Here's how the part is built. I have some questions about the finished solid (model axes, mm). Face numbers are marked on the shaded views. A direction names the side the tool comes from. Coordinates: 2 decimals unless noted, no trailing zeros. Write each loop counter-clockwise with the first axis right and the second up, starting at its lowest first coordinate (ties: lowest second). Pieces come first, ordered by that corner, then holes.
Item 1: Please list where these lines run through material, in increasing order: line 1 (Z direction, x = 16, y = 0.35); line 2 (X direction, y = 6.5, z = 10); line 3 (Y direction, x = -16.5, z = 5).
Item 2: I want a section at C-C (y = 5.75). Please give me the cut outline in (x, z).
Item 3: I want a section at B-B (x = 0). Please give me the cut outline in (y, z), and give its area (3 significant figures).
Item 4: For the marked faces 1 and 2, which set-ups out of +Z, -Z, +X, -X, +Y, -Y let a thin tool reach every point of the face, with its end or its side?
Item 5: I want a section at D-D (z = 16). Count the separate pieces of the cut face and the enclosed holes in it, and give its area (3 significant figures).
Item 6: I'm going to push flat-ended pins straight in: P1, Ø4.5, axis at x = 16, z = 16, coming from the +Y side; P2, Ø6.5, axis at x = -16, z = 16, coming from the +Y side; P3, Ø1, axis at y = 7, z = 5.5, coming from the +X side; P4, Ø10, axis at x = 11, z = -9.5, coming from the -Y side. Where does each tip first touch, or does it pass through?
Item 7: I want a section at A-A (z = 0). Please give me the cut outline in (x, y), and give its area (3 significant figures).
from build123d import *

# Parameters (mm, degrees)
ESQUISSE1_W             = 42
ESQUISSE1_H             = 42
BOSS_EXTRU_1_DEPTH      = 1
CONG_1_R                = 3
ENL_V_MAT_EXTRU_1_REACH = 11
ESQUISSE3_R             = 2


with BuildPart() as part:
    # Esquisse1 → Boss.-Extru.1 (new body)
    with BuildSketch(Plane(origin=(0, 0, 0), x_dir=(1, 0, 0), z_dir=(0, 1, 0))):
        Rectangle(ESQUISSE1_W, ESQUISSE1_H)
    extrude(amount=BOSS_EXTRU_1_DEPTH)

    # Congé1
    cong_1_edges = [part.edges().sort_by_distance(p)[0] for p in [
        (-21, 0.5, -21),
        (21, 0.5, -21),
        (21, 0.5, 21),
        (-21, 0.5, 21),
    ]]
    fillet(cong_1_edges, radius=CONG_1_R)

    # Esquisse2 → Révolution1 (revolve)
    with BuildSketch(Plane(origin=(0, 0, 0), x_dir=(0, 0, -1), z_dir=(1, 0, 0))):
        with BuildLine():
            Line((-20, 1), (-16.490388922, 3.457456133))
            ThreePointArc((-16.490388922, 3.457456133), (-15.671777012, 3.861150852), (-14.769659613, 4))
            Line((-14.769659613, 4), (-14, 4))
            Line((-14, 4), (-14, 7))
            ThreePointArc((-14, 7), (-13.414213562, 8.414213562), (-12, 9))
            Line((-12, 9), (0, 9))
            Line((0, 9), (0, 4))
            Line((0, 4), (0, 1))
            Line((0, 1), (-20, 1))
        make_face()
    revolve(axis=Axis((0, 4, 0), (0, -1, 0)))

    # Esquisse3 → Enlèv. mat.-Extru.1 (cut, up to next)
    with BuildSketch(Plane.XZ, mode=Mode.PRIVATE) as enl_v_mat_extru_1_sk1:
        with Locations((-16, 16)):
            Circle(ESQUISSE3_R)
    enl_v_mat_extru_1_tool1 = extrude(enl_v_mat_extru_1_sk1.sketch, amount=-ENL_V_MAT_EXTRU_1_REACH, mode=Mode.PRIVATE) & part.part
    add(enl_v_mat_extru_1_tool1.solids().sort_by_distance((-16, 0, 16))[0], mode=Mode.SUBTRACT)
    # Esquisse3 → Enlèv. mat.-Extru.1 (cut, up to next)
    with BuildSketch(Plane.XZ, mode=Mode.PRIVATE) as enl_v_mat_extru_1_sk2:
        with Locations((16, 16)):
            Circle(ESQUISSE3_R)
    enl_v_mat_extru_1_tool2 = extrude(enl_v_mat_extru_1_sk2.sketch, amount=-ENL_V_MAT_EXTRU_1_REACH, mode=Mode.PRIVATE) & part.part
    add(enl_v_mat_extru_1_tool2.solids().sort_by_distance((16, 0, 16))[0], mode=Mode.SUBTRACT)
    # Esquisse3 → Enlèv. mat.-Extru.1 (cut, up to next)
    with BuildSketch(Plane.XZ, mode=Mode.PRIVATE) as enl_v_mat_extru_1_sk3:
        with Locations((-16, -16)):
            Circle(ESQUISSE3_R)
    enl_v_mat_extru_1_tool3 = extrude(enl_v_mat_extru_1_sk3.sketch, amount=-ENL_V_MAT_EXTRU_1_REACH, mode=Mode.PRIVATE) & part.part
    add(enl_v_mat_extru_1_tool3.solids().sort_by_distance((-16, 0, -16))[0], mode=Mode.SUBTRACT)
    # Esquisse3 → Enlèv. mat.-Extru.1 (cut, up to next)
    with BuildSketch(Plane.XZ, mode=Mode.PRIVATE) as enl_v_mat_extru_1_sk4:
        with Locations((16, -16)):
            Circle(ESQUISSE3_R)
    enl_v_mat_extru_1_tool4 = extrude(enl_v_mat_extru_1_sk4.sketch, amount=-ENL_V_MAT_EXTRU_1_REACH, mode=Mode.PRIVATE) & part.part
    add(enl_v_mat_extru_1_tool4.solids().sort_by_distance((16, 0, -16))[0], mode=Mode.SUBTRACT)


solid = part.part
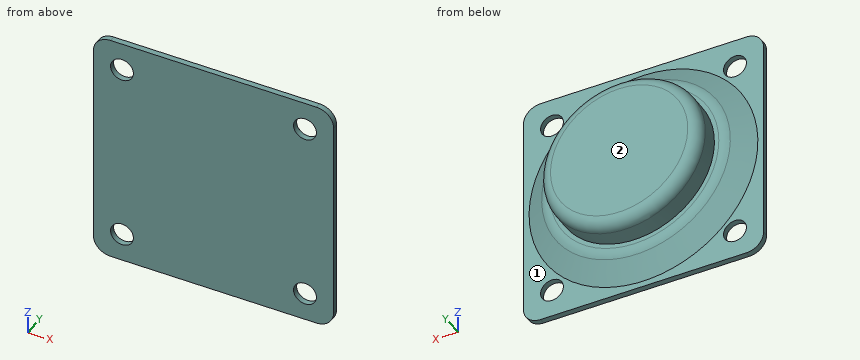
Answer:
1. line 1: z = -21 to -18, -14 to 14, 18 to 21
1. line 2: x = -9.8 to 9.8
1. line 3: y = 0 to 2.93
2. outline: circle Ø28 at (0, 0)
3. outline: (0, -21) - (1, -21) - (1, -20) - (3.46, -16.49) arc R3 ccw to (4, -14.77) - (4, -14) - (7, -14) arc R2 ccw to (9, -12) - (9, 12) arc R2 ccw to (7, 14) - (4, 14) - (4, 14.77) arc R3 ccw to (3.46, 16.49) - (1, 20) - (1, 21) - (0, 21) - close
3. area: 287 mm2
4. face 1: +Y
4. face 2: +Z, -Z, +X, -X, +Y
5. separate pieces: 3
5. enclosed holes: 0
5. area: 77.5 mm2
6. P1: stops at y = 1
6. P2: stops at y = 1.44
6. P3: stops at x = 13.08
6. P4: stops at y = 0
7. outline: (-21, 0) - (21, 0) - (21, 1) - (20, 1) - (16.49, 3.46) arc R3 ccw to (14.77, 4) - (14, 4) - (14, 7) arc R2 ccw to (12, 9) - (-12, 9) arc R2 ccw to (-14, 7) - (-14, 4) - (-14.77, 4) arc R3 ccw to (-16.49, 3.46) - (-20, 1) - (-21, 1) - close
7. area: 287 mm2
